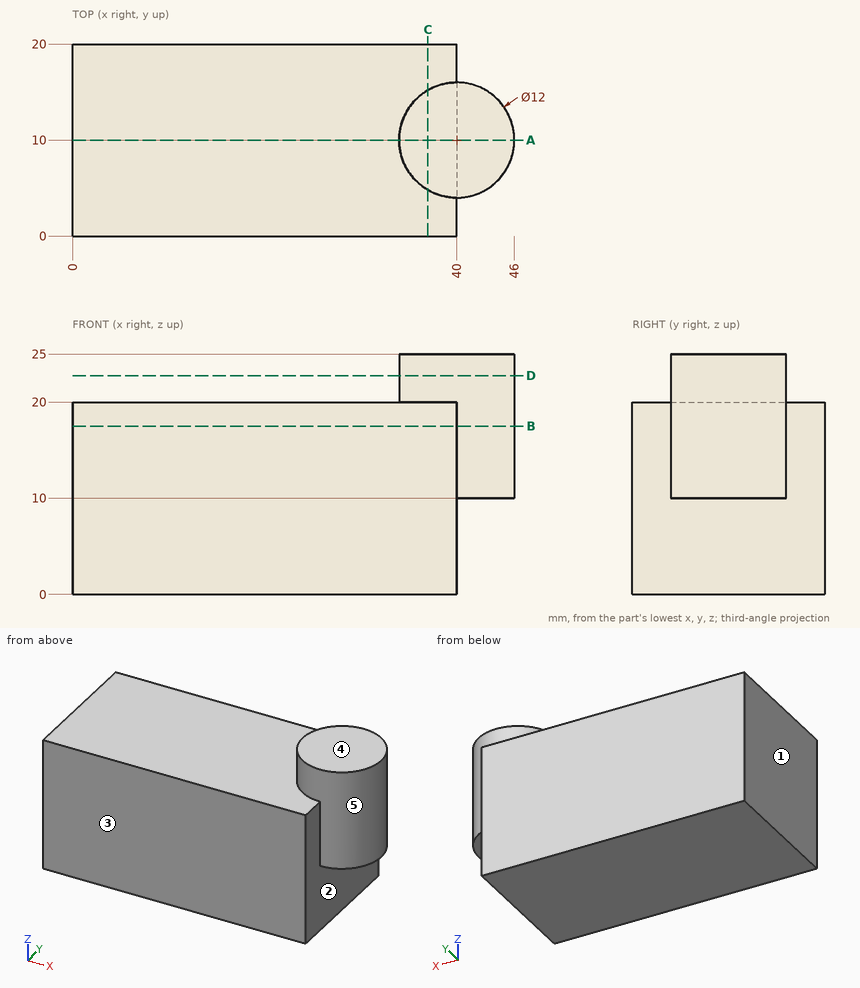
Study the drawing (mm; zero at the part's minimum x, y, z) and answer. A direction names the side the tool comes from. Round coordinates to 2 decimals unless told otherwise and drop trailing zeros. Write each loop counter-clockwise with the first axis right and the second up, starting at its lowest first coordinate (ties: lowest second). Pieces come first, ordered by that corner, then holes. Notation, with made-up numbers: (75.5, -26.5) -> (96.5, -26.5) arc R17 ccw to (96.5, 4.5) -> close; hole circle Ø2 at (79.5, 31). An arc over 180 degrees is marked (long way). Use CSV: the item, a comma, the result in double quotes. Start each with the question number.
(1) Section B-B on z = 17.5 is taken. Give the vertices of the cut face in (x, y).
(2) Which of the six approach directions +Z, -Z, +X, -X, +Y, -Y give full straight-line access (tool end or side, diameter ignored) to the marked faces 1 and 2?
(3) Section D-D on z = 22.75 is taken. Give the vertices of the cut face in (x, y), then the cut area to 3 significant figures.
(4) Section A-A on y = 10 is taken. Give the vertices of the cut face in (x, z), then the cut area to 3 significant figures.
(5) Consider L1, parallel to Z at x = 2.5, y = 6.75; L2, parallel to X at y = 6.5, z = 6; L3, parallel to Z at x = 40.5, y = 13. Determine where each line is inside the solid, lowest interval first. Write a range as from..to.
(6) Section C-C on x = 37 is taken. Give the vertices of the cut face in (y, z).
(7) The mould has two halves that part along Y. Classify the marked faces 3, 4 and 5: released by +Y, released by -Y, zero draft, split by the parting line, or undercut.
(8) Each of these flat-tipped pins is pushed along its axis until it touches: pin 1 (8 mm diameter, centred on x = 11.5, y = 15.5, fed in from -Z); pin 2 (6 mm diameter, centred on y = 6.5, z = 14.5, fed in from +X); pin 3 (10 mm diameter, centred on x = 29, y = 9, fed in from +Z). Where does it stop, or does it pass through?
A:
1,outline,"(0, 0) -> (40, 0) -> (40, 4) arc R6 ccw to (40, 16) -> (40, 20) -> (0, 20) -> close"
2,face 1,"+Z, -Z, -X, +Y, -Y"
2,face 2,"-Z, +X"
3,outline,"circle Ø12 at (40, 10)"
3,area,"113 mm²"
4,outline,"(0, 0) -> (40, 0) -> (40, 10) -> (46, 10) -> (46, 25) -> (34, 25) -> (34, 20) -> (0, 20) -> close"
4,area,"920 mm²"
5,L1,"z = 0..20"
5,L2,"x = 0..40"
5,L3,"z = 10..25"
6,outline,"(0, 0) -> (20, 0) -> (20, 20) -> (15.2, 20) -> (15.2, 25) -> (4.8, 25) -> (4.8, 20) -> (0, 20) -> close"
7,face 3,"released by -Y"
7,face 4,"zero draft"
7,face 5,"split by the parting line"
8,pin 1,"stops at z = 0"
8,pin 2,"stops at x = 45.98"
8,pin 3,"stops at z = 20"
